```python
from build123d import *

# Parameters (mm, degrees)
F0_W     = 24
F0_H     = 34
F1_DEPTH = 80
F2_R     = 10
F3_DEPTH = 25
F4_W     = 20
F4_H     = 30
F5_DEPTH = 40
F6_R     = 2.1
F7_DEPTH = 40


with BuildPart() as f1:
    # F0 (on Top) → F1 (new body)
    with BuildSketch(Plane.XY):
        with Locations((-18.134795, 17)):
            Rectangle(F0_W, F0_H)
    extrude(amount=F1_DEPTH)

    # F2 (on face) → F3 (cut)
    with BuildSketch(Plane.YZ.offset(-6.134795)):
        with Locations((17, 25)):
            Circle(F2_R)
    extrude(amount=-F3_DEPTH, mode=Mode.SUBTRACT)

    # F4 (on face) → F5 (cut)
    with BuildSketch(Plane.XY.offset(80)):
        with Locations((-18.134795, 17)):
            Rectangle(F4_W, F4_H)
    extrude(amount=-F5_DEPTH, mode=Mode.SUBTRACT)

    # F6 (on face) → F7 (cut)
    with BuildSketch(Plane(origin=(0, 34, 0), x_dir=(-1, 0, 0), z_dir=(0, 1, 0))):
        with Locations((18.134795, 70)):
            Circle(F6_R)
        with Locations((18.134795, 50)):
            Circle(F6_R)
    extrude(amount=-F7_DEPTH, mode=Mode.SUBTRACT)


solid = f1.part
```
Geometry: final body of the model. Coordinates: model frame, mm. A direction names the side the tool comes from. Coordinates: 2 decimals unless noted, no trailing zeros. Order: outer loops, then holes, each group sorted by start corner. A loop starts at its lowest first (then second) coordinate and runs counter-clockwise, first axis right, second up. Notation, with made-up numbers: (4, 36.25) - (62, 36.25) arc R30 cw to (62, 65.25) - close; hole circle Ø9 at (0.5, 53.25). An arc over 180 degrees is marked (long way). Write each question's results on one line, items separated by ' | '.
(1) Set-up query: faces 1 (the face through (-8.135, 17, 60)), 2 (the face through (-29, 17, 80)). Return all of +Z, -Z, +X, -X, +Y, -Y with unobstructed straight access to the full face (end or side cutting, diameter ignored); none if empty.
Values found:
face 1: +Z | face 2: +Z, +X, -X, +Y, -Y
(2) Section query D-D, the plane z = 58. Return the cut outline in (x, y).
Values found:
outline: (-30.13, 0) - (-6.13, 0) - (-6.13, 34) - (-30.13, 34) - close; hole (-28.13, 2) - (-8.13, 2) - (-8.13, 32) - (-28.13, 32) - close
(3) Mould query, pull axis Y, two halves, no side actions, for faces 3 (the face through (-18, 0, 39)), 4 (the face through (-17.97, 26.54, 28)), 5 (the face through (-16.47, 33.01, 68.72)), 6 (the face through (-18, 34, 39)). Classes: +Y half, -Y half, draft (parallel to the pull), parting line (faces both ways), or undercut.
Values found:
face 3: -Y half | face 4: undercut | face 5: draft | face 6: +Y half
(4) Section query A-A, the plane z = 50. Return the cut outline in (x, y).
Values found:
outline: (-30.13, 0) - (-20.23, 0) - (-20.23, 2) - (-28.13, 2) - (-28.13, 32) - (-20.23, 32) - (-20.23, 34) - (-30.13, 34) - close; (-16.03, 0) - (-6.13, 0) - (-6.13, 34) - (-16.03, 34) - (-16.03, 32) - (-8.13, 32) - (-8.13, 2) - (-16.03, 2) - close
(5) First-contact query: pin 1 Ø4 at (x, y) = (-19, 14) entering from +Z. Flat tip, straight axial feed; report the tip coordinate or a pass-through.
Values found:
pin 1: stops at z = 40
(6) Line query: line 1 (Y direction, x = -19.75, z = 75); line 2 (X direction, y = 10, z = 68); line 3 (Z direction, x = -22.5, y = 13.5). Output: solid intervals per line, ascending. Write a range as [from, to].
Values found:
line 1: y = [0, 2], [32, 34] | line 2: x = [-30.13, -28.13], [-8.13, -6.13] | line 3: z = [0, 15.63], [34.37, 40]
(7) Section query B-B, the plane x = -22.25. Return the cut outline in (y, z).
Values found:
outline: (0, 0) - (34, 0) - (34, 80) - (32, 80) - (32, 40) - (2, 40) - (2, 80) - (0, 80) - close; hole circle Ø20 at (17, 25)
(8) Section query C-C, the plane y = 17. Return the cut outline in (x, z).
Values found:
outline: (-30.13, 0) - (-6.13, 0) - (-6.13, 15) - (-30.13, 15) - close; (-30.13, 35) - (-6.13, 35) - (-6.13, 80) - (-8.13, 80) - (-8.13, 40) - (-28.13, 40) - (-28.13, 80) - (-30.13, 80) - close
